Autodesk Inventor part; units mm, degrees
ref_plane "YZ Plane" through (0, 0, 0) normal (1, 0, 0) x (0, 1, 0)
ref_plane "XZ Plane" through (0, 0, 0) normal (0, 1, 0) x (-1, 0, 0)
ref_plane "XY Plane" through (0, 0, 0) normal (0, 0, 1) x (1, 0, 0)
sketch "Sketch1" plane through (0, 0, 0) normal (0, 0, 1) x (1, 0, 0)
  line L0 (-12.7, -12.7) -> (-12.7, 12.7)
  line L1 (-12.7, 12.7) -> (12.7, 12.7)
  line L2 (12.7, 12.7) -> (12.7, -12.7)
  line L3 (12.7, -12.7) -> (-12.7, -12.7)
  line L4 (-12.7, -12.7) -> (12.7, 12.7) construction
  line L5 (-12.7, 12.7) -> (12.7, -12.7) construction
  line L6 (11.1125, 11.1125) -> (-11.1125, 11.1125)
  line L7 (-11.1125, 11.1125) -> (-11.1125, -11.1125)
  line L8 (-11.1125, -11.1125) -> (11.1125, -11.1125)
  line L9 (11.1125, -11.1125) -> (11.1125, 11.1125)
  point P0 (0, 0)
  dimension "d0" = 25.4
  dimension "d1" = 25.4
  dimension "d2" = 1.5875
extrude "Extrusion1" add sketch "Sketch1" along normal blind 609.6
sketch "Sketch2" plane through (12.7, -12.7, 0) normal (1, 0, 0) x (0, 0, -1)
  line L0 (0, 0) -> (0, 25.4)
  line L1 (0, 25.4) -> (-609.6, 25.4)
  line L2 (-609.6, 0) -> (-609.6, 25.4)
  line L3 (0, 0) -> (-609.6, 0)
  circle A0 centre (-596.9, 12.7) radius 2.5781
  circle A1 centre (-571.5, 12.7) radius 2.5781
  circle A2 centre (-546.1, 12.7) radius 2.5781
  line L4 (-304.8, 0) -> (-304.8, 25.4) construction
  circle A3 centre (-12.7, 12.7) radius 2.5781
  circle A4 centre (-38.1, 12.7) radius 2.5781
  circle A5 centre (-63.5, 12.7) radius 2.5781
  point P0 (0, 12.7)
  dimension "d5" = 5.1562
  dimension "d7" = 12.7
  dimension "d8" = 25.4
  dimension "d9" = 25.4
extrude "Extrusion2" cut sketch "Sketch2" against normal through all contours A0 | A1 | A2 | A3 | A4 | A5
sketch "Sketch5" plane through (-12.7, 12.7, 0) normal (0, 1, 0) x (1, 0, 0)
  line L0 (25.4, 0) -> (25.4, -609.6)
  line L1 (25.4, 0) -> (25.4, -223.7994)
  line L2 (25.4, -223.7994) -> (-0.9, -223.7994)
  line L3 (-0.9, -223.7994) -> (-0.9, -681.5571)
  line L4 (-0.9, -681.5571) -> (85.6151, -690.7866)
  line L5 (85.6151, -690.7866) -> (25.4, -223.7994)
  point P0 (12.7, 0)
  dimension "d15" = 223.7994
extrude "Extrusion4" cut sketch "Sketch5" against normal blind 101.6
sketch "Sketch6" plane through (12.7, -12.7, 0) normal (1, 0, 0) x (0, 0, -1)
  line L0 (-223.7994, 1.5875) -> (-223.7994, 23.8125)
  line L1 (-223.7994, 12.7) -> (-211.0994, 12.7)
  circle A0 centre (-211.0994, 12.7) radius 2.5781
  line L2 (-211.0994, 12.7) -> (-185.6994, 12.7)
  circle A1 centre (-185.6994, 12.7) radius 2.5781
  line L3 (-185.6994, 12.7) -> (-160.2994, 12.7)
  circle A2 centre (-160.2994, 12.7) radius 2.5781
  point P0 (0, 12.7)
  dimension "d18" = 12.7
  dimension "d19" = 5.1562
  dimension "d20" = 25.4
  dimension "d21" = 5.1562
  dimension "d22" = 25.4
  dimension "d23" = 5.1562
extrude "Extrusion5" cut sketch "Sketch6" against normal blind 50.8
equation "\"d1\" = d0"
properties part number "24in long 1in square tube"
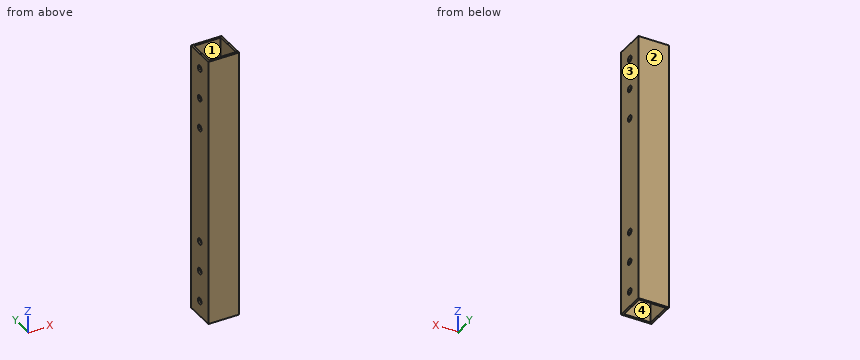
Source: CAD feature listing. Evaluate the final solid. Frame: model axes, mm. Face numbers are marked on the shaded views. Give positions to 0.01 mm unless a question says otherwise; leave off trailing zeros. Order: outer loops, then holes, each group sorted by start corner. A loop starts at its lowest first (then second) coordinate and runs counter-clockwise, first axis right, second up. Notation, with made-up numbers: (12.25, 13) -> (22.25, 13) arc R24 cw to (22.25, 36) -> close; hole circle Ø3 at (59, 58.25). An arc over 180 degrees is marked (long way). Write item = value, one per line.
Item 1: Mould query, pull axis Y, two halves, no side actions, for the marked faces 1, 2, 3 and 4. Classes: +Y half, -Y half, draft (parallel to the pull), parting line (faces both ways), or undercut.
Check result:
face_1 = undercut
face_2 = +Y half
face_3 = draft
face_4 = undercut
Item 2: Section query C-C (z = 63.5). Output: boundary loops of the cut face in (x, y).
Check result:
outline = (-12.7, -12.7) -> (12.7, -12.7) -> (12.7, -2.58) -> (11.11, -2.58) -> (11.11, -11.11) -> (-11.11, -11.11) -> (-11.11, -2.58) -> (-12.7, -2.58) -> close; (-12.7, 2.58) -> (-11.11, 2.58) -> (-11.11, 11.11) -> (11.11, 11.11) -> (11.11, 2.58) -> (12.7, 2.58) -> (12.7, 12.7) -> (-12.7, 12.7) -> close
Item 3: Ray query, probe 1 along Y at (x, z) = (7.25, 115); probe 2 along Y at (x, z) = (-12.25, 38.1). Return the intervals inside material, ascending.
Check result:
probe_1 = -12.7 to -11.11, 11.11 to 12.7
probe_2 = -12.7 to -2.58, 2.58 to 12.7
Item 4: Section query D-D (y = 0). State how many separate pieces and enclosed holes the cut face has, then the cut area to 3 significant figures.
Check result:
separate_pieces = 14
enclosed_holes = 0
area = 612 mm²
Item 5: Contact query for a flat-ended pin moving along its axis: pin 1 (3 mm diameter, centred on y = 0, z = 12.7, fed in from +X). Output: stop coordinate, or through.
Check result:
pin_1 = through
Item 6: Section query A-A (y = -9). Output: boundary loops of the cut face in (x, z), then the cut area to 3 significant figures.
Check result:
outline = (-12.7, 0) -> (-11.11, 0) -> (-11.11, 223.8) -> (-12.7, 223.8) -> close; (11.11, 0) -> (12.7, 0) -> (12.7, 223.8) -> (11.11, 223.8) -> close
area = 711 mm²
